from build123d import *

# Parameters (mm, degrees)
SKETCH_1_W                    = 25.5
SKETCH_1_H                    = 14.7
EXTRUDE_263_DEPTH             = 11.4
SKETCH_2_R                    = 1.4
EXTRUDE_429_DEPTH             = 9.8
SKETCH_3_W                    = 8.5
SKETCH_3_H                    = 5.45
SKETCH_3_R                    = 1
EXTRUDE_694_DEPTH             = 3
FILLET_3_RADIUS               = 4.25
FILLET_3_LENGTH               = 3
FILLET_3_OF_MIRROR_3_2_RADIUS = 4.25
FILLET_3_OF_MIRROR_3_2_LENGTH = 3


with BuildPart() as part:
    # 草图1 → Extrude 263 (new body)
    with BuildSketch(Plane(origin=(0, 0, 0), x_dir=(1, 0, 0), z_dir=(0, 1, 0))):
        Rectangle(SKETCH_1_W, SKETCH_1_H)
    extrude(amount=EXTRUDE_263_DEPTH)

    # 草图2 → Extrude 429 (add)
    with BuildSketch(Plane(origin=(12.75, 0, 0), x_dir=(0, 0, -1), z_dir=(1, 0, 0))):
        with Locations(Location((0, 5, 0), (0, 0, 180))):
            Circle(SKETCH_2_R)
    extrude(amount=EXTRUDE_429_DEPTH)

    # 草图3 → Extrude 694 (add)
    with BuildSketch(Plane.XZ):
        with Locations((-3.75, -10.075)):
            Rectangle(SKETCH_3_W, SKETCH_3_H)
        with Locations(Location((-3.75, -8.9, 0), (0, 0, 270))):
            Circle(SKETCH_3_R, mode=Mode.SUBTRACT)
    extrude_694 = extrude(amount=-EXTRUDE_694_DEPTH)

    # 圆角3: full round fillet: the end face becomes a half cylinder, R = half its width
    fillet_3_face = Plane((-3.75, 1.5, -12.8), x_dir=(0, 1, 0), z_dir=(0, 0, -1))  # on the end face: x along it, z out of the body
    fillet_3_slab = fillet_3_face.offset(-FILLET_3_RADIUS / 2) * Box(FILLET_3_LENGTH, 2 * FILLET_3_RADIUS, FILLET_3_RADIUS, mode=Mode.PRIVATE)  # the body's end, R deep
    fillet_3_round = Plane((-3.75, 1.5, -8.55), x_dir=(0, 0, -1), z_dir=(0, 1, 0)) * Cylinder(FILLET_3_RADIUS, FILLET_3_LENGTH, mode=Mode.PRIVATE)  # its axis R under the face
    add(fillet_3_slab - fillet_3_round, mode=Mode.SUBTRACT)

    # 镜向3: Extrude 694 across plane
    add(extrude_694.mirror(Plane.XY))

    # 圆角3 of Mirror 3 2: full round fillet: the end face becomes a half cylinder, R = half its width
    fillet_3_of_mirror_3_2_face = Plane((-3.75, 1.5, 12.8), x_dir=(0, 1, 0), z_dir=(0, 0, 1))  # on the end face: x along it, z out of the body
    fillet_3_of_mirror_3_2_slab = fillet_3_of_mirror_3_2_face.offset(-FILLET_3_OF_MIRROR_3_2_RADIUS / 2) * Box(FILLET_3_OF_MIRROR_3_2_LENGTH, 2 * FILLET_3_OF_MIRROR_3_2_RADIUS, FILLET_3_OF_MIRROR_3_2_RADIUS, mode=Mode.PRIVATE)  # the body's end, R deep
    fillet_3_of_mirror_3_2_round = Plane((-3.75, 1.5, 8.55), x_dir=(0, 0, 1), z_dir=(0, 1, 0)) * Cylinder(FILLET_3_OF_MIRROR_3_2_RADIUS, FILLET_3_OF_MIRROR_3_2_LENGTH, mode=Mode.PRIVATE)  # its axis R under the face
    add(fillet_3_of_mirror_3_2_slab - fillet_3_of_mirror_3_2_round, mode=Mode.SUBTRACT)


solid = part.part
Geometry check sheet. Reference: the model listing, model coordinates, mm. A direction names the side the tool comes from. Give positions to 0.01 mm unless a question says otherwise; leave off trailing zeros. Write each loop counter-clockwise with the first axis right and the second up, starting at its lowest first coordinate (ties: lowest second). Pieces come first, ordered by that corner, then holes. Notation, with made-up numbers: M -38,68 L -28,68 A16 ccw -28,84 Z; hole C 77,-10 d5. An arc over 180 degrees is marked long. One line per question, with ' | ' between items.
1. Mould release check, pull along X, two halves, no side actions. Record for faces 1 (the face through (12.75, 7, 0)), 2 (the face through (-4, 3, 11)), 3 (the face through (-3.7, 1.5, 7.9)): released by +X, released by -X, zero draft, split by the parting line, or undercut.
Ans:
face 1: released by +X | face 2: zero draft | face 3: undercut
2. Gauge pin test, flat ends, axial feed: pin 1 (1.2 mm diameter, centred on x = -3.75, z = 8.9, fed in from -Y); pin 2 (1 mm diameter, centred on y = 2, z = -8, fed in from +X); pin 3 (1 mm diameter, centred on y = 1.5, z = -8, fed in from -X); pin 4 (2 mm diameter, centred on y = 3, z = 2.5, fed in from +X). Record the tip position at first contact, or that the pin passes through.
Ans:
pin 1: through | pin 2: x = 0.5 | pin 3: x = -8 | pin 4: x = 12.75
3. Cross-section at C-C (y = 5). Enter the section's corners in (x, z).
Ans:
outline: M -12.75,-7.35 L 12.75,-7.35 L 12.75,-1.4 L 22.55,-1.4 L 22.55,1.4 L 12.75,1.4 L 12.75,7.35 L -12.75,7.35 Z
4. Set-up check for faces 4 (the face through (-8, 1, 8)), 5 (the face through (0.5, 1, 8)), 6 (the face through (0.5, 1, -8)), 7 (the face through (-8, 1, -8)), 8 (the face through (17.581, 6.367, -0.303)): record each of +Z, -Z, +X, -X, +Y, -Y from which the full face is reachable in a straight line by a thin tool's end or side.
Ans:
face 4: +Z, -X, +Y, -Y | face 5: +Z, +X, +Y, -Y | face 6: -Z, +X, +Y, -Y | face 7: -Z, -X, +Y, -Y | face 8: +X
5. Scan lines: line 1 along X through (y, z) = (8, 1.75); line 2 along X through (y, z) = (1.55, 8.9); line 3 along Z through (x, y) = (0, 7). Record each from-to range of solid material in increasing order. Write a range as from..to.
Ans:
line 1: -12.75..12.75 | line 2: -7.99..-4.75, -2.75..0.49 | line 3: -7.35..7.35
6. Cross-section at A-A (x = -3.75). Enter the section's corners in (y, z).
Ans:
outline: M 0,-12.8 L 3,-12.8 L 3,-9.9 L 0,-9.9 Z; M 0,-7.9 L 3,-7.9 L 3,-7.35 L 11.4,-7.35 L 11.4,7.35 L 3,7.35 L 3,7.9 L 0,7.9 Z; M 0,9.9 L 3,9.9 L 3,12.8 L 0,12.8 Z
7. Cross-section at D-D (z = 0). Enter the section's corners in (x, y), plus the area to 3 significant figures.
Ans:
outline: M -12.75,0 L 12.75,0 L 12.75,3.6 L 22.55,3.6 L 22.55,6.4 L 12.75,6.4 L 12.75,11.4 L -12.75,11.4 Z | area: 318 mm2
8. Cross-section at B-B (y = 2.25). Enter the section's corners in (x, z), plus the area to 3 significant figures.
Ans:
outline: M -12.75,-7.35 L -8,-7.35 L -8,-8.55 A4.25 ccw 0.5,-8.55 L 0.5,-7.35 L 12.75,-7.35 L 12.75,7.35 L 0.5,7.35 L 0.5,8.55 A4.25 ccw -8,8.55 L -8,7.35 L -12.75,7.35 Z; hole C -3.75,-8.9 d2; hole C -3.75,8.9 d2 | area: 446 mm2
